Geometry check sheet. Reference: the model listing, model coordinates, mm. Face numbers are marked on the shaded views. Coordinates: 2 decimals unless noted, no trailing zeros. Write each loop counter-clockwise with the first axis right and the second up, starting at its lowest first coordinate (ties: lowest second). Pieces come first, ordered by that corner, then holes. Notation, with made-up numbers: M 34.5,29.25 L 71.5,29.25 A28 ccw 71.5,67.25 Z; hole C -40,-38.5 d7. An arc over 180 degrees is marked long. Answer as a JSON object with one key per item and string values. Group by question number.
```python
from build123d import *

# Parameters (mm, degrees)
SKETCH1_R                = 25
SKETCH1_R_2              = 20.015
BOSS_EXTRUDE1_DEPTH      = 50
BOSS_EXTRUDE2_DEPTH      = 50
FILLET1_R                = 2
CIRPATTERN1_COUNT        = 6
FILLET1_OF_CIRPATTERN1_R = 2


with BuildPart() as part:
    # Sketch1 → Boss-Extrude1 (new body)
    with BuildSketch(Plane.XY):
        Circle(SKETCH1_R)
        Circle(SKETCH1_R_2, mode=Mode.SUBTRACT)
    extrude(amount=-BOSS_EXTRUDE1_DEPTH)

    # Sketch2 → Boss-Extrude2 (add)
    with BuildSketch(Plane.XY):
        with BuildLine():
            Line((6.470476128, 24.148145657), (7.764571353, 28.977774789))
            ThreePointArc((7.764571353, 28.977774789), (0, 30), (-7.764571353, 28.977774789))
            Line((-7.764571353, 28.977774789), (-6.470476128, 24.148145657))
            ThreePointArc((-6.470476128, 24.148145657), (0, 25), (6.470476128, 24.148145657))
        make_face()
    boss_extrude2 = extrude(amount=-BOSS_EXTRUDE2_DEPTH)

    # Fillet1
    fillet1_edges = [part.edges().sort_by_distance(p)[0] for p in [
        (-7.764571353, 28.977774789, -25),
        (7.764571353, 28.977774789, -25),
    ]]
    fillet(fillet1_edges, radius=FILLET1_R)

    # CirPattern1: Boss-Extrude2 ×6 about axis
    cirpattern1_axis = Axis((0, 0, 0), (0, 0, 1))
    for i in range(1, CIRPATTERN1_COUNT):
        add(boss_extrude2.rotate(cirpattern1_axis, i * 360 / CIRPATTERN1_COUNT))

    # Fillet1 of CirPattern1
    fillet1_of_cirpattern1_edges = [part.edges().sort_by_distance(p)[0] for p in [
        (-28.977774789, 7.764571353, -25),
        (-21.213203436, 21.213203436, -25),
        (-21.213203436, -21.213203436, -25),
        (-28.977774789, -7.764571353, -25),
        (7.764571353, -28.977774789, -25),
        (-7.764571353, -28.977774789, -25),
        (28.977774789, -7.764571353, -25),
        (21.213203436, -21.213203436, -25),
        (21.213203436, 21.213203436, -25),
        (28.977774789, 7.764571353, -25),
    ]]
    fillet(fillet1_of_cirpattern1_edges, radius=FILLET1_OF_CIRPATTERN1_R)


solid = part.part
```
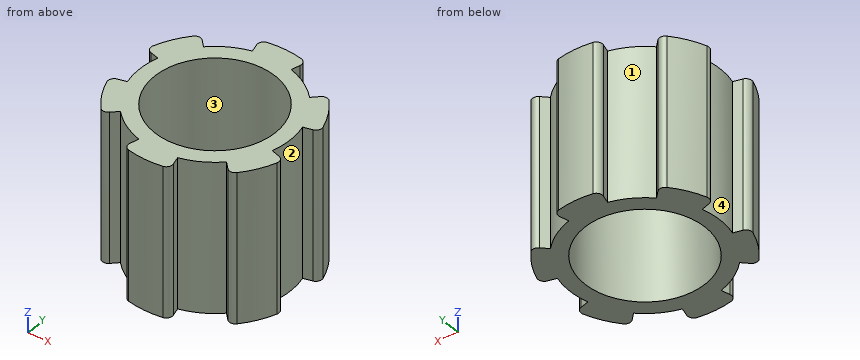
1) Section check A-A (y = 0). Record the cut outline in (x, z) (3 decimals).
2) Go/stop test with flat-tipped pins: pin 1 Ø1 at (y, z) = (-15, -7.5) entering from -X; pin 2 Ø6 at (y, z) = (15, -11.5) entering from +X; pin 3 Ø10 at (x, z) = (-22.5, -34) entering from +Y. Record where each tip stops, or that it passes through.
3) Draft check along X on the marked faces 1, 2, 3 and 4. Enter one of: +X half, -X half, draft (parallel to the pull), parting line (faces both ways), or undercut.
4) Material ranges on probe 1 along Y at (x, z) = (0, -10) (3 decimals); probe 2 along Y at (x, z) = (14.5, -23.5); probe 3 along X at (y, z) = (14.5, -21.5), recorded low to high. Write a range as [from, to].
5) Section check B-B (x = 0). Record the cut outline in (y, z) (3 decimals), then the cut area to 4 significant figures.
Entries:
{
 "1": {"outline": "M -25,-50 L -20.015,-50 L -20.015,0 L -25,0 Z; M 20.015,-50 L 25,-50 L 25,0 L 20.015,0 Z"},
 "2": {"pin 1": "x = -26.26", "pin 2": "x = 27.5", "pin 3": "y = 20.33"},
 "3": {"face 1": "undercut", "face 2": "+X half", "face 3": "undercut", "face 4": "-X half"},
 "4": {"probe 1": "[-30, -20.015], [20.015, 30]", "probe 2": "[-20.37, -13.8], [13.8, 20.37]", "probe 3": "[-26.26, -13.8], [13.8, 26.26]"},
 "5": {"outline": "M -30,-50 L -20.015,-50 L -20.015,0 L -30,0 Z; M 20.015,-50 L 30,-50 L 30,0 L 20.015,0 Z", "area": "998.5 mm^2"}
}
